```python
from build123d import *

# Parameters (mm, degrees)
SKETCH1_W           = 60
SKETCH1_H           = 130
BOSS_EXTRUDE1_DEPTH = 5
SKETCH2_W           = 20
SKETCH2_H           = 15
CUT_EXTRUDE1_DEPTH  = 5
CUT_EXTRUDE2_DEPTH  = 5


with BuildPart() as part:
    # Sketch1 → Boss-Extrude1 (new body)
    with BuildSketch(Plane.XY):
        Rectangle(SKETCH1_W, SKETCH1_H)
    extrude(amount=BOSS_EXTRUDE1_DEPTH)

    # Sketch2 → Cut-Extrude1 (cut)
    with BuildSketch(Plane(origin=(0, 0, 0), x_dir=(-1, 0, 0), z_dir=(0, 0, -1))):
        with Locations((0, -30)):
            Rectangle(SKETCH2_W, SKETCH2_H)
    extrude(amount=-CUT_EXTRUDE1_DEPTH, mode=Mode.SUBTRACT)

    # Sketch3 → Cut-Extrude2 (cut)
    with BuildSketch(Plane(origin=(0, 0, 0), x_dir=(-1, 0, 0), z_dir=(0, 0, -1))):
        with BuildLine():
            Line((16.8, -25), (16.8, -35))
            ThreePointArc((16.8, -35), (15, -36.8), (13.2, -35))
            Line((13.2, -35), (13.2, -25))
            ThreePointArc((13.2, -25), (15, -23.2), (16.8, -25))
        make_face()
        with BuildLine():
            Line((-13.2, -25), (-13.2, -35))
            ThreePointArc((-13.2, -35), (-15, -36.8), (-16.8, -35))
            Line((-16.8, -35), (-16.8, -25))
            ThreePointArc((-16.8, -25), (-15, -23.2), (-13.2, -25))
        make_face()
    extrude(amount=-CUT_EXTRUDE2_DEPTH, mode=Mode.SUBTRACT)


solid = part.part
```
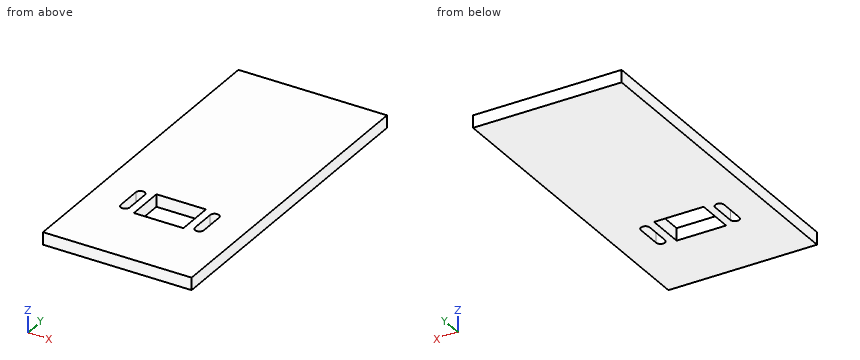
Read the model definition and answer for the solid it produces. Units are mm, in the model's axes. Give positions to 0.01 mm unless a question says otherwise; leave off trailing zeros. Write each loop counter-clockwise with the first axis right and the second up, starting at its lowest first coordinate (ties: lowest second). Pieces come first, ordered by that corner, then holes. Notation, with made-up numbers: (28.5, 43.25) - (87.5, 43.25) arc R18 ccw to (87.5, 47.25) - close; hole circle Ø7 at (-37.5, 63.25). An arc over 180 degrees is marked (long way). Write item = value, one per line. Start each with the question number.
Item 1: This flat-tipped pin is pushed along its axis until it touches: P1, Ø5, axis at x = -21.5, y = -43, coming from the -Z side. Where does it stop, or does it pass through?
Item 2: Find section A-A (z = 0.85). Give the vertices of the cut face in (x, y), then the cut area to 3 significant figures.
Item 3: Find section B-B (x = -15). Give the vertices of the cut face in (y, z), then the cut area to 3 significant figures.
Item 4: Find the intervals of material crossed by probe 1 along X at (y, z) = (-32, 1.1); probe 2 along Y at (x, z) = (-2, 1.7); probe 3 along Y at (x, z) = (-14, 3.3), in increasing order. Write a range as [from, to].
Item 5: Find section C-C (x = 0). Give the vertices of the cut face in (y, z), then the cut area to 3 significant figures.
Response:
q1.P1 = 0
q2.outline = (-30, -65) - (30, -65) - (30, 65) - (-30, 65) - close; hole (-16.8, -35) arc R1.8 ccw to (-13.2, -35) - (-13.2, -25) arc R1.8 ccw to (-16.8, -25) - close; hole (-10, -37.5) - (10, -37.5) - (10, -22.5) - (-10, -22.5) - close; hole (13.2, -35) arc R1.8 ccw to (16.8, -35) - (16.8, -25) arc R1.8 ccw to (13.2, -25) - close
q2.area = 7,410 mm²
q3.outline = (-65, 0) - (-36.8, 0) - (-36.8, 5) - (-65, 5) - close; (-23.2, 0) - (65, 0) - (65, 5) - (-23.2, 5) - close
q3.area = 582 mm²
q4.probe_1 = [-30, -16.8], [-13.2, -10], [10, 13.2], [16.8, 30]
q4.probe_2 = [-65, -37.5], [-22.5, 65]
q4.probe_3 = [-65, -36.5], [-23.5, 65]
q5.outline = (-65, 0) - (-37.5, 0) - (-37.5, 5) - (-65, 5) - close; (-22.5, 0) - (65, 0) - (65, 5) - (-22.5, 5) - close
q5.area = 575 mm²
